Geometry: final body of the model. Coordinates: model frame, mm. A direction names the side the tool comes from. Give positions to 0.01 mm unless a question says otherwise; leave off trailing zeros. Write each loop counter-clockwise with the first axis right and the second up, starting at its lowest first coordinate (ties: lowest second). Pieces come first, ordered by that corner, then holes.
Q1. Draft query along Y for faces 1 (the face through (-8.3, 5.5, 0.4)), 2 (the face through (-5.5, 7, 0)), 3 (the face through (2, 0, 1)), 4 (the face through (2, 12.2, -1)). Return one class per face: pulls with the +Y half, pulls with the -Y half, needs draft (parallel to the pull), parting line crosses it, or undercut.
Q2. Cut plane B-B on x = 0. Return the cut outline in (y, z).
Q3. Line query: L1, parallel to Y at x = -7.5, z = 0; L2, parallel to X at y = 13.6, z = 0; L3, parallel to X at y = 7.75, z = 0. Output: solid intervals per line, ascending.
Q4. Pin query (flat end, axial travel): pin 1 (5 mm diameter, centred on y = 7, z = -4, fed in from -X); pin 2 (2.5 mm diameter, centred on y = 7.1, z = 0, fed in from +X); pin 3 (5.5 mm diameter, centred on x = 0, z = 0, fed in from +Y). Return the tip coordinate at first contact, or that it passes through.
Q5. Cut plane A-A on z = 0. Return the cut outline in (x, y), plus the area to 3 significant figures.
Q6. Reachability of faces 5 (the face through (10.85, 6.95, 2.41)), 6 (the face through (8.3, 5.5, 0.4)), 7 (the face through (-0.9, -1.01, -2.86)), 8 (the face through (2.3, 14.2, -2.3)) from +Z, -Z, +X, -X, +Y, -Y: full face, straight path, thin tool, end or side. Return the list, or none.
Q7. Cut plane C-C on x = 6.5. Return the cut outline in (y, z).
```python
from build123d import *

# Parameters (mm, degrees)
CUT_EXTRUDE1_REACH      = 30.396
CUT_EXTRUDE1_END_RADIUS = 11.1125
CUT_EXTRUDE1_START      = -5.5
SKETCH2_R               = 1.65


with BuildPart() as part:
    # Sketch1 → Revolve1 (revolve)
    with BuildSketch(Plane(origin=(0, 0, 0), x_dir=(0, 0, -1), z_dir=(1, 0, 0)), mode=Mode.PRIVATE) as revolve1_sk:
        Polygon((-2, 0), (-3, 0), (-3, -2), (-12.7, -2), (-12.7, -0.5), (-11.1125, -0.5), (-11.1125, 14.2), (-3, 14.2), (-3, 12.2), (-2, 12.2), align=None)
    revolve(revolve1_sk.sketch.rotate(Axis((0, -1000, 0), (0, 1, 0)), 180), axis=Axis((0, -1000, 0), (0, 1, 0)))

    # Cut-Extrude1: up to this cylinder (the profile starts inside it)
    cut_extrude1_end = Plane(origin=(0, 7.1, 0), z_dir=(0, -1, 0)) * Cylinder(CUT_EXTRUDE1_END_RADIUS, 84.017, mode=Mode.PRIVATE)
    # Sketch2 → Cut-Extrude1 (cut, up to the surface)
    with BuildSketch(Plane(origin=(0, 0, 0), x_dir=(0, 0, -1), z_dir=(1, 0, 0)).offset(CUT_EXTRUDE1_START), mode=Mode.PRIVATE) as cut_extrude1_sk1:
        with Locations((0, 7.1)):
            Circle(SKETCH2_R)
    cut_extrude1_tool1 = extrude(cut_extrude1_sk1.sketch, amount=-CUT_EXTRUDE1_REACH, mode=Mode.PRIVATE) & cut_extrude1_end
    cut_extrude1 = cut_extrude1_tool1.solids().sort_by_distance((-5.5, 7.1, 0))[0]
    add(cut_extrude1, mode=Mode.SUBTRACT)

    # Mirror1: Cut-Extrude1 across plane
    add(cut_extrude1.mirror(Plane(origin=(0, 0, 0), x_dir=(0, 0, 1), z_dir=(1, 0, 0))), mode=Mode.SUBTRACT)


solid = part.part
```
Data:
1. face 1: undercut
1. face 2: undercut
1. face 3: pulls with the -Y half
1. face 4: pulls with the +Y half
2. outline: (-2, -12.7) - (-0.5, -12.7) - (-0.5, -11.11) - (14.2, -11.11) - (14.2, -3) - (12.2, -3) - (12.2, -2) - (0, -2) - (0, -3) - (-2, -3) - close; (-2, 3) - (0, 3) - (0, 2) - (12.2, 2) - (12.2, 3) - (14.2, 3) - (14.2, 11.11) - (-0.5, 11.11) - (-0.5, 12.7) - (-2, 12.7) - close
3. L1: y = -2 to 5.45, 8.75 to 14.2
3. L2: x = -11.11 to -3, 3 to 11.11
3. L3: x = -5.5 to -2, 2 to 5.5
4. pin 1: stops at x = -11
4. pin 2: stops at x = 5.5
4. pin 3: stops at y = 12.2
5. outline: (-12.7, -2) - (-3, -2) - (-3, 0) - (-2, 0) - (-2, 12.2) - (-3, 12.2) - (-3, 14.2) - (-11.11, 14.2) - (-11.11, 8.75) - (-5.5, 8.75) - (-5.5, 5.45) - (-11.11, 5.45) - (-11.11, -0.5) - (-12.7, -0.5) - close; (2, 0) - (3, 0) - (3, -2) - (12.7, -2) - (12.7, -0.5) - (11.11, -0.5) - (11.11, 5.45) - (5.5, 5.45) - (5.5, 8.75) - (11.11, 8.75) - (11.11, 14.2) - (3, 14.2) - (3, 12.2) - (2, 12.2) - close
5. area: 255 mm2
6. face 5: +Y
6. face 6: +X
6. face 7: -Y
6. face 8: +Z, -Z, +X, -X, +Y
7. outline: (-2, -10.91) - (-0.5, -10.91) - (-0.5, -9.01) - (14.2, -9.01) - (14.2, 9.01) - (-0.5, 9.01) - (-0.5, 10.91) - (-2, 10.91) - close; hole circle Ø3.3 at (7.1, 0)
